```python
from build123d import *

# Parameters (mm, degrees)
SKETCH1_R           = 2.286
SKETCH1_R_2         = 1.905
BOSS_EXTRUDE1_DEPTH = 18.796
SKETCH2_W           = 44.45
SKETCH2_H           = 6.604
CUT_EXTRUDE1_DEPTH  = 43.179298429
SKETCH3_R           = 4.445
CUT_EXTRUDE2_DEPTH  = 2.54
BOSS_EXTRUDE2_START = -6.096
SKETCH4_R           = 2.286
SKETCH4_R_2         = 1.905
BOSS_EXTRUDE2_DEPTH = 6.096
FILLET1_R           = 3.81


with BuildPart() as part:
    # Sketch1 → Boss-Extrude1 (new body)
    with BuildSketch(Plane(origin=(0, 0, 0), x_dir=(1, 0, 0), z_dir=(0, 1, 0))):
        with BuildLine():
            Line((-29.21, 6.35), (29.21, 6.35))
            ThreePointArc((29.21, 6.35), (35.56, 0), (29.21, -6.35))
            Line((29.21, -6.35), (-29.21, -6.35))
            ThreePointArc((-29.21, -6.35), (-35.56, 0), (-29.21, 6.35))
        make_face()
        with Locations(Location((-29.21, 0, 0), (0, 0, 270))):
            Circle(SKETCH1_R, mode=Mode.SUBTRACT)
        with Locations(Location((29.21, 0, 0), (0, 0, 270))):
            Circle(SKETCH1_R_2, mode=Mode.SUBTRACT)
    extrude(amount=BOSS_EXTRUDE1_DEPTH)

    # Sketch2 → Cut-Extrude1 (cut, through all)
    with BuildSketch(Plane.XY.offset(6.35)):
        with Locations((-13.335, 9.398)):
            Rectangle(SKETCH2_W, SKETCH2_H)
    extrude(amount=-CUT_EXTRUDE1_DEPTH, mode=Mode.SUBTRACT)

    # Sketch3 → Cut-Extrude2 (cut)
    with BuildSketch(Plane(origin=(0, 18.796, 0), x_dir=(1, 0, 0), z_dir=(0, 1, 0))):
        with Locations(Location((-29.21, 0, 0), (0, 0, 270))):
            Circle(SKETCH3_R)
    extrude(amount=-CUT_EXTRUDE2_DEPTH, mode=Mode.SUBTRACT)

    # Sketch4 → Boss-Extrude2 (add)
    with BuildSketch(Plane(origin=(0, 6.096, 0), x_dir=(1, 0, 0), z_dir=(0, 1, 0)).offset(BOSS_EXTRUDE2_START)):
        with Locations(Location((-29.21, 0, 0), (0, 0, 270))):
            Circle(SKETCH4_R)
        with Locations(Location((-29.21, 0, 0), (0, 0, 180))):
            Circle(SKETCH4_R_2, mode=Mode.SUBTRACT)
    extrude(amount=BOSS_EXTRUDE2_DEPTH)

    # Fillet1
    fillet1_edges = [part.edges().sort_by_distance(p)[0] for p in [
        (8.89, 9.398, 6.35),
        (8.89, 9.398, -6.35),
    ]]
    fillet(fillet1_edges, radius=FILLET1_R)


solid = part.part
```
Design review of the part built by this model. Coordinates are the model's own, in mm. A direction names the side the tool comes from. Give positions to 0.01 mm unless a question says otherwise; leave off trailing zeros. Loops run counter-clockwise (first coordinate to the right, second up) from the corner with the lowest first, then second, coordinate; pieces in that order, holes last. Notation, with made-up numbers: (15.5, 16.5) -> (34.5, 16.5) arc R24 ccw to (34.5, 40.5) -> close; hole circle Ø8 at (22, 27). An arc over 180 degrees is marked (long way). One line per item, written item: value.
Q1. We need section C-C on z = 0. Give the boundary of the cut face in (x, y) (3 decimals), and give its area (3 significant figures).
Numbers:
outline: (-35.56, 0) -> (-31.115, 0) -> (-31.115, 6.096) -> (-35.56, 6.096) -> close; (-35.56, 12.7) -> (-31.496, 12.7) -> (-31.496, 16.256) -> (-33.655, 16.256) -> (-33.655, 18.796) -> (-35.56, 18.796) -> close; (-27.305, 0) -> (27.305, 0) -> (27.305, 18.796) -> (-24.765, 18.796) -> (-24.765, 16.256) -> (-26.924, 16.256) -> (-26.924, 12.7) -> (8.89, 12.7) -> (8.89, 6.096) -> (-27.305, 6.096) -> close; (31.115, 0) -> (35.56, 0) -> (35.56, 18.796) -> (31.115, 18.796) -> close
area: 910 mm^2
Q2. Draft analysis for pull direction Z (two halves, no side actions). For faces 6 (the flat face through (0, 5, -6.35)), 7 (the cylindrical face through (-24.803, 17.544, -0.579)), 8 (the flat face through (0, 18.796, 0)), state which applies: pulls with the +Z half, pulls with the -Z half, needs draft (parallel to the pull), parting line crosses it, or undercut.
Numbers:
face 6: pulls with the -Z half
face 7: undercut
face 8: needs draft
Q3. We need section B-B on x = -22. Give the boundary of the cut face in (y, z), and give its area (3 significant figures).
Numbers:
outline: (0, -6.35) -> (6.1, -6.35) -> (6.1, 6.35) -> (0, 6.35) -> close; (12.7, -6.35) -> (18.8, -6.35) -> (18.8, 6.35) -> (12.7, 6.35) -> close
area: 155 mm^2
Q4. We need section A-A on y = 7. Give the boundary of the cut face in (x, z) (3 decimals).
Numbers:
outline: (8.89, -2.54) arc R3.81 ccw to (12.7, -6.35) -> (29.21, -6.35) arc R6.35 ccw to (29.21, 6.35) -> (12.7, 6.35) arc R3.81 ccw to (8.89, 2.54) -> close; hole circle Ø3.81 at (29.21, 0)
Q5. For L1, parallel to X at y = 17.4, z = 0 (3 decimals); L2, parallel to X at y = 14, z = 0 (3 decimals); L3, parallel to Y at x = -8, z = 2.75, list the stretches that pass through material, from the lowest coordinate up.
Numbers:
L1: x = -35.56 to -33.655, -24.765 to 27.305, 31.115 to 35.56
L2: x = -35.56 to -31.496, -26.924 to 27.305, 31.115 to 35.56
L3: y = 0 to 6.1, 12.7 to 18.8
Q6. We need section D-D on y = 3.5. Give the boundary of the cut face in (x, z) (3 decimals).
Numbers:
outline: (-29.21, -6.35) -> (29.21, -6.35) arc R6.35 ccw to (29.21, 6.35) -> (-29.21, 6.35) arc R6.35 ccw to start; hole circle Ø3.81 at (-29.21, 0); hole circle Ø3.81 at (29.21, 0)
Q7. For pin 1 Ø1.5 at (y, z) = (9, 3) entering from +X; pin 2 Ø3.5 at (x, z) = (-29.21, 0) entering from -Y; pin 3 Ø1.5 at (y, z) = (4.5, 2.5) entering from -X; pin 4 Ø7 at (x, z) = (-29.21, 0) entering from +Y, all flat-tipped, find the tip position at first contact; note any pin that passes through.
Numbers:
pin 1: stops at x = 35.15
pin 2: passes through
pin 3: stops at x = -35.31
pin 4: stops at y = 16.26
Q8. Machinability: for faces 1 (the flat face through (-31, 16.256, 2)), 2 (the cylindrical face through (10.036, 9.352, -5.264)), 3 (the flat face through (0, 5, 6.35)), 4 (the flat face through (8.89, 9, 0)), 5 (the cylindrical face through (10.036, 9.444, 5.264)), which of the approach directions +Z, -Z, +X, -X, +Y, -Y give a long, thin tool a straight path to every point of the face, cutting with its end or side? Answer none if there is none.
Numbers:
face 1: +Y
face 2: -Z, -X
face 3: +Z, +X, -X, +Y, -Y
face 4: +Z, -Z, -X
face 5: +Z, -X
